Read the model definition and answer for the solid it produces. Units are mm, in the model's axes. Face numbers are marked on the shaded views. A direction names the side the tool comes from. Give positions to 0.01 mm unless a question says otherwise; leave off trailing zeros. Write each loop counter-clockwise with the first axis right and the second up, starting at its lowest first coordinate (ties: lowest second). Pieces come first, ordered by that corner, then holes.
```python
from build123d import *

# Parameters (mm, degrees)
ESBO_O3_W                = 90
ESBO_O3_H                = 50
RESSALTO_EXTRUS_O1_DEPTH = 10


with BuildPart() as part:
    # Esboço3 → Ressalto-extrusão1 (new body)
    with BuildSketch(Plane.XY):
        with Locations((45, 25)):
            Rectangle(ESBO_O3_W, ESBO_O3_H)
        with BuildLine():
            Line((9.25, 46), (20.75, 46))
            ThreePointArc((20.75, 46), (24.75, 42), (20.75, 38))
            Line((20.75, 38), (9.25, 38))
            ThreePointArc((9.25, 38), (5.25, 42), (9.25, 46))
        make_face(mode=Mode.SUBTRACT)
        with BuildLine():
            Line((80.75, 38), (69.25, 38))
            ThreePointArc((69.25, 38), (65.25, 42), (69.25, 46))
            Line((69.25, 46), (80.75, 46))
            ThreePointArc((80.75, 46), (84.75, 42), (80.75, 38))
        make_face(mode=Mode.SUBTRACT)
        with BuildLine():
            Line((9.25, 12), (20.75, 12))
            ThreePointArc((20.75, 12), (24.75, 8), (20.75, 4))
            Line((20.75, 4), (9.25, 4))
            ThreePointArc((9.25, 4), (5.25, 8), (9.25, 12))
        make_face(mode=Mode.SUBTRACT)
        with BuildLine():
            Line((69.25, 12), (80.75, 12))
            ThreePointArc((80.75, 12), (84.75, 8), (80.75, 4))
            Line((80.75, 4), (69.25, 4))
            ThreePointArc((69.25, 4), (65.25, 8), (69.25, 12))
        make_face(mode=Mode.SUBTRACT)
    extrude(amount=RESSALTO_EXTRUS_O1_DEPTH)


solid = part.part
```
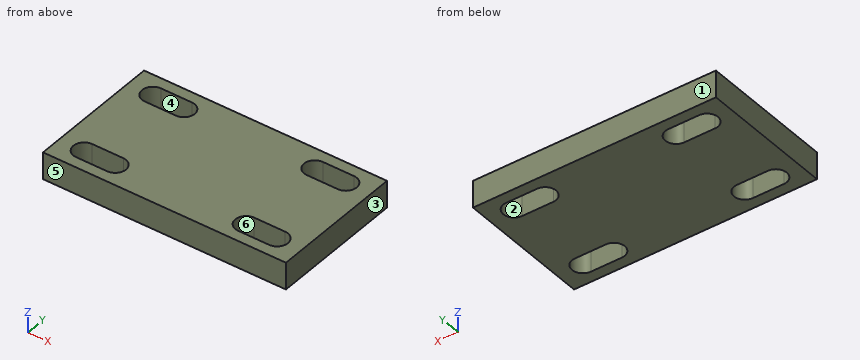
Item 1: Which of the six approach directions +Z, -Z, +X, -X, +Y, -Y give full straight-line access (tool end or side, diameter ignored) to the marked faces 5 and 6?
Result set:
face 5: +Z, -Z, +X, -X, -Y
face 6: +Z, -Z
Item 2: Find the intervals of material crossed by line 1 along Y through (x, z) = (17, 4.5); line 2 along X through (y, z) = (40.5, 8.5); line 3 along X through (y, z) = (40, 7.75), in increasing order.
Result set:
line 1: y = 0 to 4, 12 to 38, 46 to 50
line 2: x = 0 to 5.54, 24.46 to 65.54, 84.46 to 90
line 3: x = 0 to 5.79, 24.21 to 65.79, 84.21 to 90
Item 3: Section C-C (y = 5) is taken. Write down the section's boundary in (x, z).
Result set:
outline: (0, 0) - (6.6, 0) - (6.6, 10) - (0, 10) - close; (23.4, 0) - (66.6, 0) - (66.6, 10) - (23.4, 10) - close; (83.4, 0) - (90, 0) - (90, 10) - (83.4, 10) - close
Item 4: Section A-A (x = 14.5) is taken. Write down the section's boundary in (y, z).
Result set:
outline: (0, 0) - (4, 0) - (4, 10) - (0, 10) - close; (12, 0) - (38, 0) - (38, 10) - (12, 10) - close; (46, 0) - (50, 0) - (50, 10) - (46, 10) - close
Item 5: Determine the mould class of the marked faces 1, 2, 3 and 4 for opening direction Y: pulls with the +Y half, pulls with the -Y half, needs draft (parallel to the pull), parting line crosses it, or undercut.
Result set:
face 1: pulls with the +Y half
face 2: undercut
face 3: needs draft
face 4: undercut
Item 6: Section B-B (z = 6) is taken. Write down the section's boundary in (x, y).
Result set:
outline: (0, 0) - (90, 0) - (90, 50) - (0, 50) - close; hole (9.25, 4) - (20.75, 4) arc R4 ccw to (20.75, 12) - (9.25, 12) arc R4 ccw to start; hole (9.25, 38) - (20.75, 38) arc R4 ccw to (20.75, 46) - (9.25, 46) arc R4 ccw to start; hole (69.25, 4) - (80.75, 4) arc R4 ccw to (80.75, 12) - (69.25, 12) arc R4 ccw to start; hole (69.25, 38) - (80.75, 38) arc R4 ccw to (80.75, 46) - (69.25, 46) arc R4 ccw to start
